from build123d import *

# Parameters (mm, degrees)
F0_R     = 7
F0_R_2   = 2.5
F1_DEPTH = 5
F2_R     = 6
F2_R_2   = 3.5
F3_DEPTH = 0.25
F4_R     = 6
F4_R_2   = 3.5
F5_DEPTH = 0.25
F6_R     = 0.2


with BuildPart() as f1:
    # F0 (on Right) → F1 (new body)
    with BuildSketch(Plane.YZ):
        Circle(F0_R)
        Circle(F0_R_2, mode=Mode.SUBTRACT)
    extrude(amount=F1_DEPTH)

    # F2 (on Right) → F3 (cut)
    with BuildSketch(Plane.YZ):
        Circle(F2_R)
        Circle(F2_R_2, mode=Mode.SUBTRACT)
    extrude(amount=F3_DEPTH, mode=Mode.SUBTRACT)

    # F4 (on face) → F5 (cut)
    with BuildSketch(Plane.YZ.offset(5)):
        Circle(F4_R)
        Circle(F4_R_2, mode=Mode.SUBTRACT)
    extrude(amount=-F5_DEPTH, mode=Mode.SUBTRACT)

    # F6
    f6_edges = [f1.edges().sort_by_distance(p)[0] for p in [
        (2.5, 7, 0),
        (0, -7, 0),
        (5, -7, 0),
        (2.5, 2.5, 0),
        (0, -2.5, 0),
        (5, -2.5, 0),
    ]]
    fillet(f6_edges, radius=F6_R)


solid = f1.part
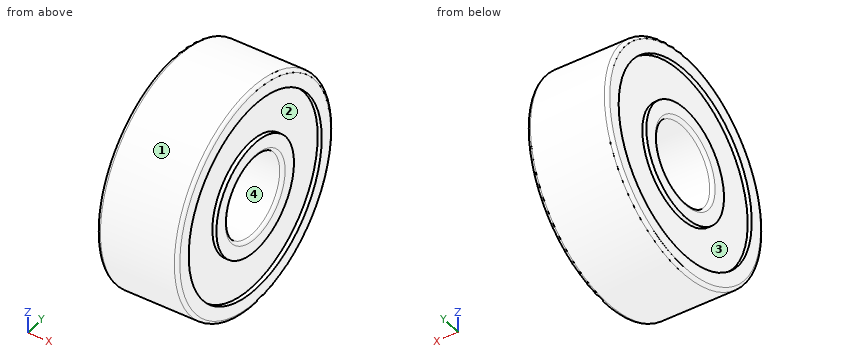
Here's how the part is built. I have some questions about the finished solid (model axes, mm). Face numbers are marked on the shaded views. A direction names the side the tool comes from. Coordinates: 2 decimals unless noted, no trailing zeros. Write each loop counter-clockwise with the first axis right and the second up, starting at its lowest first coordinate (ties: lowest second). Pieces come first, ordered by that corner, then holes.
Item 1: If we mould it in two halves opening along Y, with no side actions, what happens to the marked faces 1 and 2? For each: +Y half, -Y half, draft (parallel to the pull), parting line (faces both ways), or undercut.
Item 2: Will these pins go through, and if not, where does the flat tip stop? pin 1 (1 mm diameter, centred on x = 2, y = 5, fed in from -Z); pin 2 (1.5 mm diameter, centred on x = 0.5, y = -5, fed in from -Z); pin 3 (1 mm diameter, centred on x = 3, z = 1.5, fed in from +Y).
Item 3: I want a section at C-C on x = 1.7. Write out the boundary of the cut face in (y, z).
Item 4: If I drill on line 1 (Z direction, x = 4.9, y = 0); line 2 (Z direction, x = 1.5, y = -1); line 3 (X direction, y = -5.25, z = -2.25), over which ranges is the centre line in solid material (lowest first)?
Item 5: On a 3-axis mill with a long thin cutter (end or side, diameter ignored), from which of +Z, -Z, +X, -X, +Y, -Y can I reach the whole of each face in a straight line? I mean the marked faces 3 and 4. Say none if no direction works.
Findings below:
1. face 1: parting line
1. face 2: undercut
2. pin 1: stops at z = -5.36
2. pin 2: stops at z = -5.56
2. pin 3: stops at y = 6.93
3. outline: circle Ø14 at (0, 0); hole circle Ø5 at (0, 0)
4. line 1: z = -6.97 to -6, -3.5 to -2.53, 2.53 to 3.5, 6 to 6.97
4. line 2: z = -6.93 to -2.29, 2.29 to 6.93
4. line 3: x = 0.25 to 4.75
5. face 3: -X
5. face 4: +X, -X
